from build123d import *

# Parameters (mm, degrees)
SKETCH1_R           = 31.5
SKETCH1_R_2         = 26
BOSS_EXTRUDE1_DEPTH = 35
SKETCH1_3_R         = 18
SKETCH1_3_R_2       = 12
BOSS_EXTRUDE2_DEPTH = 21
BOSS_EXTRUDE3_DEPTH = 21
BOSS_EXTRUDE4_DEPTH = 7
SKETCH2_R           = 5
BOSS_EXTRUDE5_DEPTH = 7
CUT_EXTRUDE6_START  = -21
CUT_EXTRUDE6_DEPTH  = 42
SKETCH1_7_R         = 18
SKETCH1_7_R_2       = 12
BOSS_EXTRUDE6_DEPTH = 21


with BuildPart() as part:
    # Sketch1 → Boss-Extrude1 (new, symmetric)
    with BuildSketch(Plane.YZ):
        with Locations(Location((0, 0, 0), (0, 0, 270))):
            Circle(SKETCH1_R)
        with Locations(Location((0, 0, 0), (0, 0, 270))):
            Circle(SKETCH1_R_2, mode=Mode.SUBTRACT)
    extrude(amount=BOSS_EXTRUDE1_DEPTH, both=True)



with BuildPart() as body_2:
    # Sketch1<3> → Boss-Extrude2 (new, symmetric)
    with BuildSketch(Plane.YZ):
        with Locations(Location((250, 0, 0), (0, 0, 90))):
            Circle(SKETCH1_3_R)
        with Locations(Location((250, 0, 0), (0, 0, 90))):
            Circle(SKETCH1_3_R_2, mode=Mode.SUBTRACT)
    extrude(amount=BOSS_EXTRUDE2_DEPTH, both=True)


with BuildPart() as part_1:
    add(part.part)

    add(body_2.part)  # Boss-Extrude3 merges body 2
    # Sketch1<4> → Boss-Extrude3 (add, symmetric)
    with BuildSketch(Plane.YZ):
        with BuildLine():
            Line((235.379808483, 10.5), (88, 21))
            Line((88, 21), (23.478713764, 21))
            ThreePointArc((23.478713764, 21), (29.426429307, 11.239895828), (31.5, 0))
            ThreePointArc((31.5, 0), (29.426429307, -11.239895828), (23.478713764, -21))
            Line((23.478713764, -21), (88, -21))
            Line((88, -21), (235.379808483, -10.5))
            ThreePointArc((235.379808483, -10.5), (232, 0), (235.379808483, 10.5))
        make_face()
        with BuildLine():
            ThreePointArc((70, -6), (64, 0), (70, 6))
            Line((70, 6), (220, 6))
            ThreePointArc((220, 6), (226, 0), (220, -6))
            Line((220, -6), (70, -6))
        make_face(mode=Mode.SUBTRACT)
    extrude(amount=BOSS_EXTRUDE3_DEPTH, both=True)

    # Sketch1<5> → Boss-Extrude4 (add, symmetric)
    with BuildSketch(Plane.YZ):
        with BuildLine():
            Line((70, -6), (220, -6))
            ThreePointArc((220, -6), (226, 0), (220, 6))
            Line((220, 6), (70, 6))
            ThreePointArc((70, 6), (64, 0), (70, -6))
        make_face()
    extrude(amount=BOSS_EXTRUDE4_DEPTH, both=True)

    # Sketch2 → Boss-Extrude5 (add)
    with BuildSketch(Plane.YZ.offset(21)):
        with BuildLine():
            ThreePointArc((25.516398298, -50.647058824), (51.072598285, -28.838439215), (83.742065952, -21))
            Line((83.742065952, -21), (23.478713764, -21))
            ThreePointArc((23.478713764, -21), (-31.5, 0), (23.478713764, 21))
            Line((23.478713764, 21), (83.742065952, 21))
            ThreePointArc((83.742065952, 21), (51.072598285, 28.838439215), (25.516398298, 50.647058824))
            ThreePointArc((25.516398298, 50.647058824), (16.869455228, 55.865378029), (7.0962671, 53.318757993))
            ThreePointArc((7.0962671, 53.318757993), (-14.501700837, 41.975317571), (-38.64781523, 38.495228582))
            ThreePointArc((-38.64781523, 38.495228582), (-49.375786098, 33.332181232), (-51.401209618, 21.6))
            ThreePointArc((-51.401209618, 21.6), (-48.08483212, 0), (-51.401209618, -21.6))
            ThreePointArc((-51.401209618, -21.6), (-49.375786098, -33.332181232), (-38.64781523, -38.495228582))
            ThreePointArc((-38.64781523, -38.495228582), (-14.501700837, -41.975317571), (7.0962671, -53.318757993))
            ThreePointArc((7.0962671, -53.318757993), (16.869455228, -55.865378029), (25.516398298, -50.647058824))
        make_face()
        with Locations(Location((15.003430528, -43, 0), (0, 0, 270))):
            Circle(SKETCH2_R, mode=Mode.SUBTRACT)
        with Locations(Location((-39, -25.5, 0), (0, 0, 270))):
            Circle(SKETCH2_R, mode=Mode.SUBTRACT)
        with Locations(Location((-39, 25.5, 0), (0, 0, 270))):
            Circle(SKETCH2_R, mode=Mode.SUBTRACT)
        with Locations(Location((15.003430528, 43, 0), (0, 0, 270))):
            Circle(SKETCH2_R, mode=Mode.SUBTRACT)
    boss_extrude5 = extrude(amount=-BOSS_EXTRUDE5_DEPTH)

    # Mirror1: Boss-Extrude5 across plane
    add(boss_extrude5.mirror(Plane(origin=(0, 0, 0), x_dir=(0, 0, 1), z_dir=(1, 0, 0))))

    # Cut-Extrude6: read off the stored shape, not the designer's step
    # Cut-Extrude6 outline → Cut-Extrude6 (cut)
    with BuildSketch(Plane(origin=(0, 0, 0), x_dir=(0, 1, 0), z_dir=(0, 0, 1)).offset(CUT_EXTRUDE6_START)):
        with BuildLine():
            ThreePointArc((88, 21), (104.014282256, 15.028577262), (120.984845005, 13))
            Line((120.984845005, 13), (235.379808483, 13))
            Line((235.379808483, 13), (235.379808483, 21))
            Line((235.379808483, 21), (88, 21))
        make_face()
    cut_extrude6 = extrude(amount=CUT_EXTRUDE6_DEPTH, mode=Mode.SUBTRACT)

    # Mirror2: Cut-Extrude6 across plane
    add(cut_extrude6.mirror(Plane(origin=(0, 0, 0), x_dir=(0, 0, 1), z_dir=(1, 0, 0))), mode=Mode.SUBTRACT)

    # Sketch1<7> → Boss-Extrude6 (add, symmetric)
    with BuildSketch(Plane.YZ):
        with Locations(Location((250, 0, 0), (0, 0, 270))):
            Circle(SKETCH1_7_R)
        with Locations(Location((250, 0, 0), (0, 0, 90))):
            Circle(SKETCH1_7_R_2, mode=Mode.SUBTRACT)
    extrude(amount=BOSS_EXTRUDE6_DEPTH, both=True)


solid = part_1.part
Source: CAD feature listing. Evaluate the final solid. Frame: model axes, mm. A direction names the side the tool comes from. Round coordinates to 2 decimals unless told otherwise and drop trailing zeros. Loops run counter-clockwise (first coordinate to the right, second up) from the corner with the lowest first, then second, coordinate; pieces in that order, holes last.
Q1. Mould query, pull axis Y, two halves, no side actions, for faces 4 (the face through (17.549, 16.726, -55.885)), 5 (the face through (-17.549, 51.496, 28.624)), 6 (the face through (-11, 127, 6)), 7 (the face through (11, 127, 6)). Classes: pulls with the +Y half, pulls with the -Y half, needs draft (parallel to the pull), parting line crosses it, or undercut.
Q2. Section C-C, the plane x = 17. Return loops of the section in (y, z), plus the area to 3 significant figures.
Q3. First-contact query: P1, Ø7, axis at x = -15, y = 130, coming from the +Z side; P2, Ø13, axis at y = 15, z = 43, coming from the +X side; P3, Ø8, axis at x = -15, z = 33, coming from the -Y side. Flat tips, straight axial feed; report the tip coordinate or a pass-through.
Q4. Section A-A, the plane y = 250. Return loops of the section in (x, z).
Q5. Ray query, line 1 (Y direction, x = 2, z = 0); line 2 (X direction, y = 33, z = -33.5); line 3 (Y direction, x = 16, z = 0). Return the intervals inside material, ascending.
Q6. Section D-D, the plane z = 0. State how many separate pieces and enclosed holes the cut face has, plus the area to 3 significant figures.
Q7. Access query for faces 1 (the face through (15.085, 103.781, -13.605)), 2 (the face through (21, 254, -12)), 3 (the face through (21, 33, 1)). Directions: +Z, -Z, +X, -X, +Y, -Y. A direction counts if a zero-diameter tool reaches every point of the face in a straight line with its end or side. Return the directions, or none.
Q8. Section B-B, the plane z = -35. Return loops of the section in (x, y).
Solutions:
1. face 4: parting line crosses it
1. face 5: pulls with the +Y half
1. face 6: undercut
1. face 7: undercut
2. outline: (-51.4, -21.6) arc R13 ccw to (-38.65, -38.5) arc R72 cw to (7.1, -53.32) arc R13 ccw to (25.52, -50.65) arc R72 cw to (83.74, -21) - (88, -21) - (97.32, -20.34) - (97.32, -6) - (70, -6) arc R6 cw to (70, 6) - (97.32, 6) - (97.32, 20.34) - (88, 21) - (83.74, 21) arc R72 cw to (25.52, 50.65) arc R13 ccw to (7.1, 53.32) arc R72 cw to (-38.65, 38.5) arc R13 ccw to (-51.4, 21.6) arc R72 cw to start; circle Ø36 at (250, 0); hole circle Ø10 at (-39, -25.5); hole circle Ø10 at (-39, 25.5); hole circle Ø52 at (0, 0); hole circle Ø10 at (15, -43); hole circle Ø10 at (15, 43); hole circle Ø24 at (250, 0)
2. area: 8,570 mm2
3. P1: stops at z = 18.21
3. P2: stops at x = 21
3. P3: stops at y = -51.52
4. outline: (-21, -18) - (21, -18) - (21, -12) - (-21, -12) - close; (-21, 12) - (21, 12) - (21, 18) - (-21, 18) - close
5. line 1: y = -31.5 to -26, 26 to 238, 262 to 268
5. line 2: x = -21 to -14, 14 to 21
5. line 3: y = -48.08 to -26, 26 to 64, 232 to 238, 262 to 268
6. separate pieces: 3
6. enclosed holes: 0
6. area: 5,300 mm2
7. face 1: +Z, -Z, +X
7. face 2: +Z, -Z, +X, +Y
7. face 3: +X
8. outline: (-21, -47.87) - (-14, -47.87) - (-14, 41.08) - (-21, 41.08) - close; (14, -47.87) - (21, -47.87) - (21, 41.08) - (14, 41.08) - close
